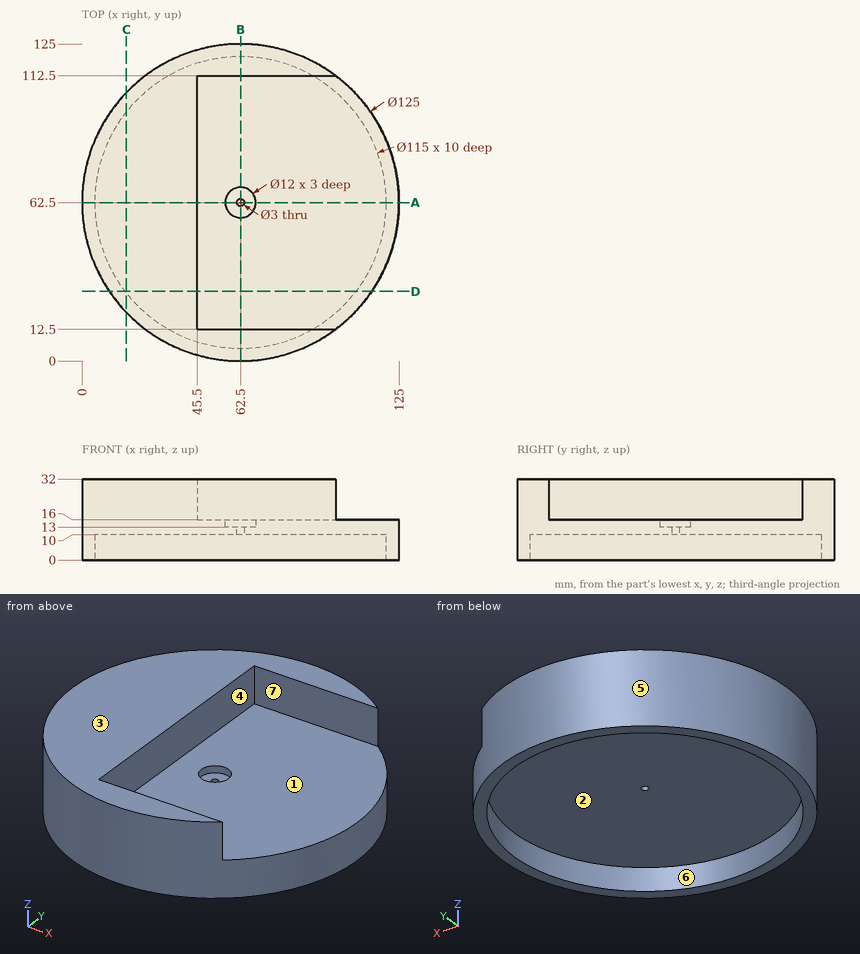
The figure shows three views and two pictorial views of one solid part (mm, origin at its lowest corner). Answer the questions. A direction names the side the tool comes from. Round coordinates to 2 decimals unless told otherwise and drop trailing zeros. Write each loop counter-clockwise with the first axis right and the second up, starting at its lowest first coordinate (ties: lowest second). Pieces come first, ordered by that corner, then holes. Notation, with made-up numbers: (-12, 18.25) - (44, 18.25) arc R19 cw to (44, 25.25) - close; hole circle Ø4 at (31.5, -36.75). An arc over 180 degrees is marked (long way). One line per question, with ' | ' between items. Start each with the question number.
1. For a pull along X with two mould halves and no side action, classify the marked faces 4, 5, 6 and 7 as +X half, -X half, draft (parallel to the pull), parting line (faces both ways), or undercut.
2. Section C-C (x = 17.5) is taken. Determine the outline of the cut face in (y, z), and give its area (3 significant figures).
3. Find the intervals of material crossed by probe 1 along Y at (x, z) = (62.5, 2.5); probe 2 along Y at (x, z) = (62.5, 12), in increasing order. Write a range as [from, to].
4. Section D-D (y = 27.5) is taken. Determine the outline of the cut face in (x, z).
5. Section B-B (x = 62.5) is taken. Determine the outline of the cut face in (y, z), and give its area (4 significant figures).
6. Section A-A (y = 62.5) is taken. Determine the outline of the cut face in (x, z), and give its area (3 significant figures).
7. Each of these flat-tipped pins is pushed along its axis until it touches: pin 1 (3.5 mm diameter, centred on x = 62.5, y = 62.5, fed in from +Z); pin 2 (5 mm diameter, centred on x = 59, z = 22, fed in from -Y); pin 3 (13 mm diameter, centred on x = 63.5, y = 62, fed in from +Z). Where does it stop, or does it pass through?
8. For the marked faces 1, 2 and 3, determine the directions among +Z, -Z, +X, -X, +Y, -Y from which every point of the face is accessible in a straight line to the end or side of a thin tool.
Filled in:
1) face 4: +X half | face 5: parting line | face 6: undercut | face 7: draft
2) outline: (19.13, 0) - (26.71, 0) - (26.71, 10) - (98.29, 10) - (98.29, 0) - (105.87, 0) - (105.87, 32) - (19.13, 32) - close | area: 2,060 mm²
3) probe 1: [0, 5], [120, 125] | probe 2: [0, 61], [64, 125]
4) outline: (10.72, 0) - (16.88, 0) - (16.88, 10) - (108.12, 10) - (108.12, 0) - (114.28, 0) - (114.28, 16) - (45.5, 16) - (45.5, 32) - (10.72, 32) - close
5) outline: (0, 0) - (5, 0) - (5, 10) - (61, 10) - (61, 13) - (56.5, 13) - (56.5, 16) - (12.5, 16) - (12.5, 32) - (0, 32) - close; (64, 10) - (120, 10) - (120, 0) - (125, 0) - (125, 32) - (112.5, 32) - (112.5, 16) - (68.5, 16) - (68.5, 13) - (64, 13) - close | area: 1,205 mm²
6) outline: (0, 0) - (5, 0) - (5, 10) - (61, 10) - (61, 13) - (56.5, 13) - (56.5, 16) - (45.5, 16) - (45.5, 32) - (0, 32) - close; (64, 10) - (120, 10) - (120, 0) - (125, 0) - (125, 16) - (68.5, 16) - (68.5, 13) - (64, 13) - close | area: 1,530 mm²
7) pin 1: z = 13 | pin 2: y = 0.01 | pin 3: z = 16
8) face 1: +Z, +X | face 2: -Z | face 3: +Z, +X, -X, +Y, -Y
